Study the drawing (mm; zero at the part's minimum x, y, z) and answer. A direction names the side the tool comes from. Round coordinates to 2 decimals unless told otherwise and drop trailing zeros. Write each loop counter-clockwise with the first axis right and the second up, starting at its lowest first coordinate (ties: lowest second). Pieces come first, ordered by that corner, then holes. Notation, with made-up numbers: M 82.25,-34 L 115.25,-34 A25 cw 115.25,-2 Z; hole C 7.5,67.25 d8. An arc over 180 degrees is marked long. Write each question's results on one line, items separated by ' | '.
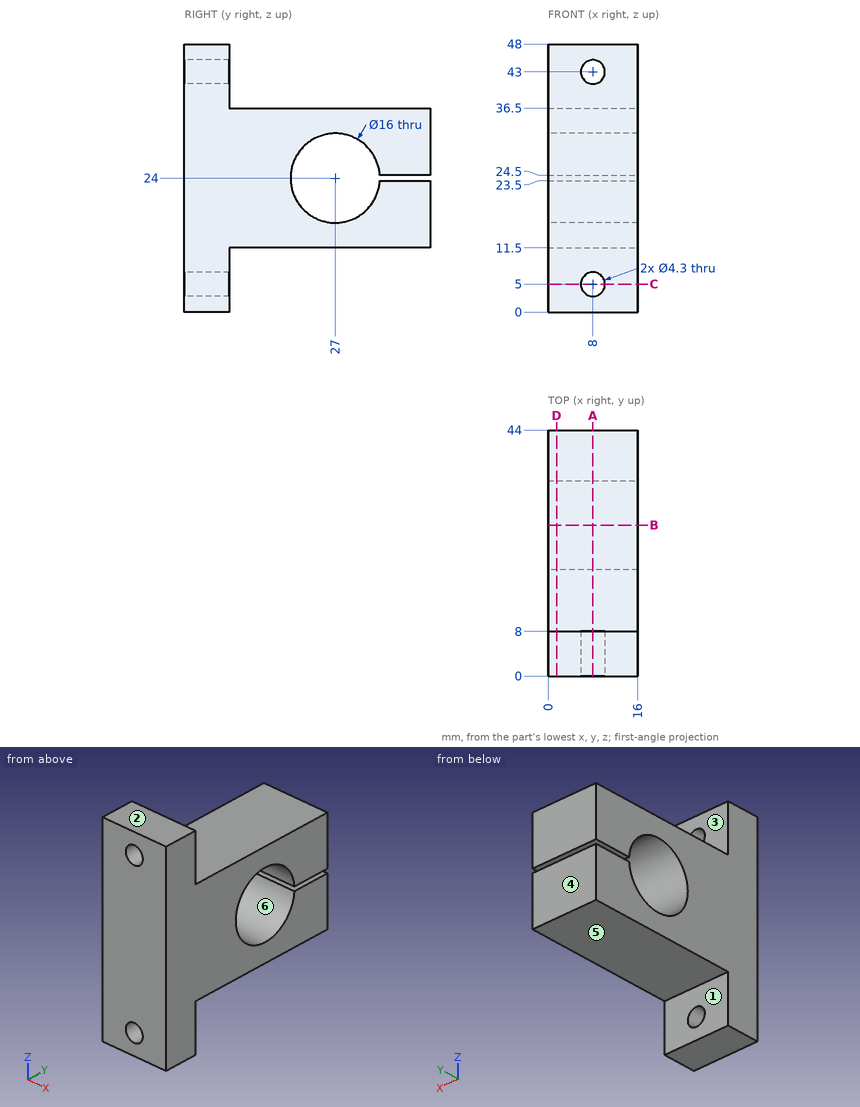
1) Section A-A (x = 8) is taken. Determine the outline of the cut face in (y, z).
Return value:
outline: M 0,0 L 8,0 L 8,2.85 L 0,2.85 Z; M 0,7.15 L 8,7.15 L 8,11.5 L 44,11.5 L 44,23.5 L 34.98,23.5 A8 cw long 34.98,24.5 L 44,24.5 L 44,36.5 L 8,36.5 L 8,40.85 L 0,40.85 Z; M 0,45.15 L 8,45.15 L 8,48 L 0,48 Z
2) The mould has two halves that part along Y. Classify the marked faces 4, 5 and 6: +Y half, -Y half, draft (parallel to the pull), parting line (faces both ways), or undercut.
Return value:
face 4: +Y half | face 5: draft | face 6: undercut
3) Section D-D (x = 1.5) is taken. Determine the outline of the cut face in (y, z), then the cut area to 3 significant figures.
Return value:
outline: M 0,0 L 8,0 L 8,11.5 L 44,11.5 L 44,23.5 L 34.98,23.5 A8 cw long 34.98,24.5 L 44,24.5 L 44,36.5 L 8,36.5 L 8,48 L 0,48 Z | area: 1,070 mm²
4) Section B-B (y = 27) is taken. Determine the outline of the cut face in (x, z).
Return value:
outline: M 0,11.5 L 16,11.5 L 16,16 L 0,16 Z; M 0,32 L 16,32 L 16,36.5 L 0,36.5 Z
5) Find the intervals of material crossed by line 1 (Z direction, x = 8, y = 3.5); line 2 (Z direction, x = 11.75, y = 27); line 3 (Z direction, x = 12.5, y = 41.5), in increasing order.
Return value:
line 1: 0 to 2.85, 7.15 to 40.85, 45.15 to 48 | line 2: 11.5 to 16, 32 to 36.5 | line 3: 11.5 to 23.5, 24.5 to 36.5
6) A tool of negligible diameter and unlimited length cuts with its end or side. For the marked faces 1, 2 and 3, from which of +Z, -Z, +X, -X, +Y, -Y can it reach the whole face along a straight path? Write none if from no direction.
Return value:
face 1: -Z, +X, -X, +Y | face 2: +Z, +X, -X, +Y, -Y | face 3: +Z, +X, -X, +Y
7) Section C-C (z = 5) is taken. Determine the outline of the cut face in (x, y).
Return value:
outline: M 0,0 L 5.85,0 L 5.85,8 L 0,8 Z; M 10.15,0 L 16,0 L 16,8 L 10.15,8 Z
8) Each of these flat-tipped pins is pushed along its axis until it touches: pin 1 (8 mm diameter, centred on x = 5, y = 17.5, fed in from +Z); pin 2 (1 mm diameter, centred on x = 9.5, y = 36, fed in from -Z); pin 3 (4 mm diameter, centred on x = 13.5, z = 10, fed in from -Y); pin 4 (6 mm diameter, centred on x = 10.5, z = 41, fed in from +Y). Where does it stop, or does it pass through?
Return value:
pin 1: z = 36.5 | pin 2: z = 11.5 | pin 3: y = 0 | pin 4: y = 8
